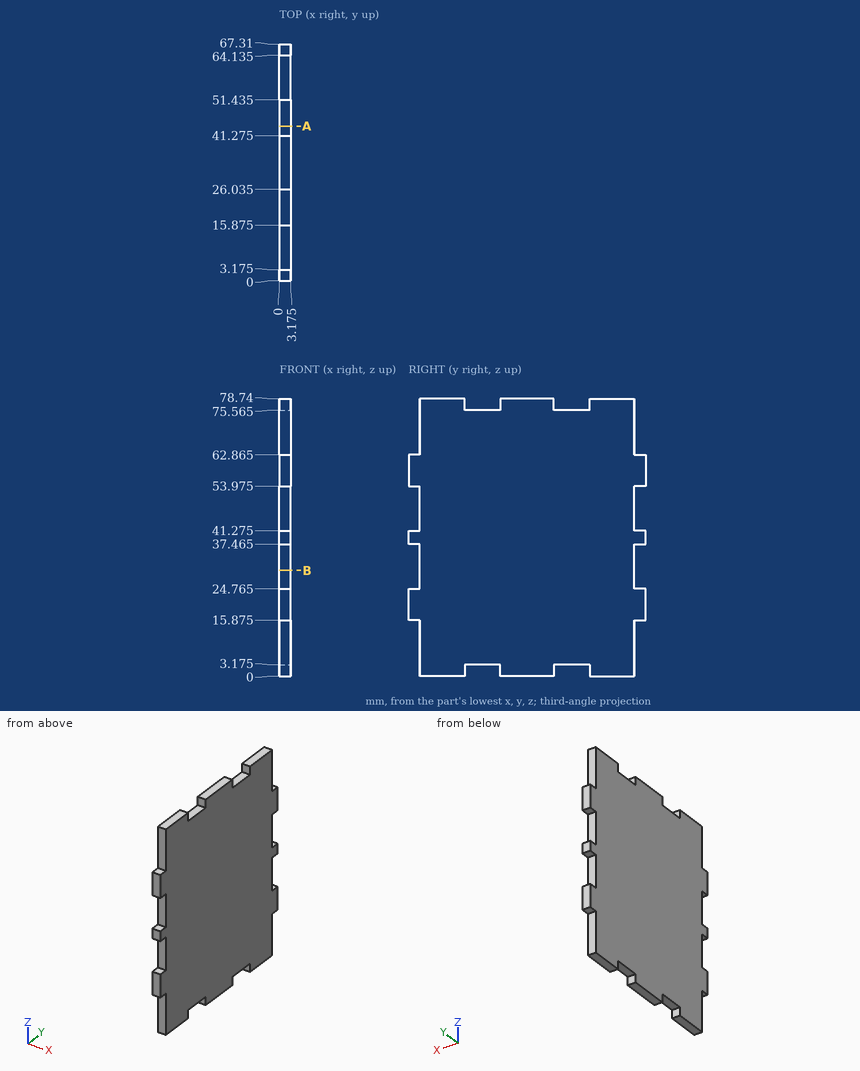
Input: dimensioned drawing with shaded views. Units: mm. Origin: part minimum x, y, z. Round coordinates to 2 decimals unless told otherwise and drop trailing zeros. Order: outer loops, then holes, each group sorted by start corner. A loop starts at its lowest first (then second) coordinate and runs counter-clockwise, first axis right, second up. Notation, with made-up numbers: (7, 39) - (62, 39) arc R33 cw to (62, 77) - close; hole circle Ø2 at (24.25, 31.25). An arc over 180 degrees is marked (long way). Answer as a JSON object with one key per item and string values. Group by question number.
(1) Pin query (flat end, axial travel): P1, Ø1, axis at x = 1.5, z = 32, coming from the +Y side (3 decimals); P2, Ø1.6, axis at x = 2, z = 45, coming from the -Y side (3 decimals); P3, Ø1.6, axis at x = 1, y = 2, coming from the -Z side (3 decimals). Return the tip coordinate at first contact, or that it passes through.
(2) Cut plane B-B (z = 30). Return loops of the section in (x, y) (3 decimals).
(3) Cut plane A-A (y = 44). Return loops of the section in (x, z) (3 decimals).
(4) Material intervals for probe 1 along Z at (x, y) = (0.9, 3) (3 decimals); probe 2 along Z at (x, y) = (1.2, 41.5) (3 decimals); probe 3 along Y at (x, z) = (2.95, 6.5) (3 decimals), sorted ascending. Write a range as from..to.
Here are the results:
{
 "1": {"P1": "stops at y = 64.135", "P2": "stops at y = 3.175", "P3": "stops at z = 15.875"},
 "2": {"outline": "(0, 3.175) - (3.175, 3.175) - (3.175, 64.135) - (0, 64.135) - close"},
 "3": {"outline": "(0, 3.175) - (3.175, 3.175) - (3.175, 75.565) - (0, 75.565) - close"},
 "4": {"probe 1": "z = 15.875..24.765, 37.465..41.275, 53.975..62.865", "probe 2": "z = 3.175..75.565", "probe 3": "y = 3.175..64.135"}
}
